from build123d import *

# Parameters (mm, degrees)
SKETCH1_R               = 6.35
BOSS_EXTRUDE1_DEPTH     = 25.4
SKETCH2_R               = 2.5
CUT_EXTRUDE1_DEPTH      = 12.7
SKETCH3_R               = 3.175
CUT_EXTRUDE2_DEPTH      = 12.7
CUT_EXTRUDE4_REACH      = 28.941
CUT_EXTRUDE4_END_RADIUS = 6.35
SKETCH4_R               = 1.3890625


with BuildPart() as part:
    # Sketch1 → Boss-Extrude1 (new body)
    with BuildSketch(Plane.XY):
        Circle(SKETCH1_R)
    extrude(amount=BOSS_EXTRUDE1_DEPTH)

    # Sketch2 → Cut-Extrude1 (cut)
    with BuildSketch(Plane.XY.offset(25.4)):
        Circle(SKETCH2_R)
    extrude(amount=-CUT_EXTRUDE1_DEPTH, mode=Mode.SUBTRACT)

    # Sketch3 → Cut-Extrude2 (cut)
    with BuildSketch(Plane(origin=(0, 0, 0), x_dir=(-1, 0, 0), z_dir=(0, 0, -1))):
        Circle(SKETCH3_R)
    extrude(amount=-CUT_EXTRUDE2_DEPTH, mode=Mode.SUBTRACT)

    # Cut-Extrude4: up to this cylinder (the profile starts inside it)
    cut_extrude4_end = Plane(origin=(0, 0, 12.7), z_dir=(0, 0, -1)) * Cylinder(CUT_EXTRUDE4_END_RADIUS, 90.632, mode=Mode.PRIVATE)
    # Sketch4 → Cut-Extrude4 (cut, up to the surface)
    with BuildSketch(Plane(origin=(0, 0, 0), x_dir=(1, 0, 0), z_dir=(0, 1, 0)), mode=Mode.PRIVATE) as cut_extrude4_sk1:
        with Locations(Location((0, -22.225, 0), (0, 0, 270))):
            Circle(SKETCH4_R)
    cut_extrude4_tool1 = extrude(cut_extrude4_sk1.sketch, amount=-CUT_EXTRUDE4_REACH, mode=Mode.PRIVATE) & cut_extrude4_end
    add(cut_extrude4_tool1.solids().sort_by_distance((0, 0, 22.225))[0], mode=Mode.SUBTRACT)
    # Sketch4 → Cut-Extrude4 (cut, up to the surface)
    with BuildSketch(Plane(origin=(0, 0, 0), x_dir=(1, 0, 0), z_dir=(0, 1, 0)), mode=Mode.PRIVATE) as cut_extrude4_sk2:
        with Locations(Location((0, -3.175, 0), (0, 0, 270))):
            Circle(SKETCH4_R)
    cut_extrude4_tool2 = extrude(cut_extrude4_sk2.sketch, amount=-CUT_EXTRUDE4_REACH, mode=Mode.PRIVATE) & cut_extrude4_end
    add(cut_extrude4_tool2.solids().sort_by_distance((0, 0, 3.175))[0], mode=Mode.SUBTRACT)


solid = part.part
Check sheet for the modelled part. Datum: model origin and axes. Units: mm. A direction names the side the tool comes from. Round coordinates to 2 decimals unless told otherwise and drop trailing zeros. Loops run counter-clockwise (first coordinate to the right, second up) from the corner with the lowest first, then second, coordinate; pieces in that order, holes last. Notation, with made-up numbers: M -25.5,70 L 3.5,70 A16 ccw 3.5,89 Z; hole C 59.5,-15.5 d10. An arc over 180 degrees is marked long. One line per question, with ' | ' between items. Start each with the question number.
Item 1: Section check C-C (z = 8.5). Record the boundary of the cut face in (x, y) (3 decimals).
Item 2: Section check A-A (y = 0). Record the boundary of the cut face in (x, z) (3 decimals).
Item 3: Gauge pin test, flat ends, axial feed: pin 1 Ø1.5 at (y, z) = (-4, 21.5) entering from -X; pin 2 Ø4 at (x, y) = (0, 0) entering from -Z; pin 3 Ø2 at (y, z) = (-3.5, 6) entering from -X. Record the tip position at first contact, or that the pin passes through.
Item 4: Section check B-B (x = 0). Record the boundary of the cut face in (y, z) (3 decimals), and give its area (3 significant figures).
Item 5: Set-up check for faces 1 (the face through (-2, 3, 0)), 2 (the face through (0.42, -4.19, 23.55)), 3 (the face through (0, -3, 12.7)): record each of +Z, -Z, +X, -X, +Y, -Y from which the full face is reachable in a straight line by a thin tool's end or side.
Item 6: Scan lines: probe 1 along Z at (x, y) = (0, -4); probe 2 along Y at (x, z) = (0, 18); probe 3 along Y at (x, z) = (0, 5.75) (3 decimals). Record each from-to range of solid material in increasing order.
Item 7: Release check for a two-part mould opening along Y. For faces 4 (the face through (-0.33, 2.48, 19.14)), 5 (the face through (-1.38, -6.2, 12.52)), 6 (the face through (0.41, 3.15, 6.26)), 7 (the face through (0.42, -4.58, 4.5)) record: released by +Y, released by -Y, zero draft, split by the parting line, or undercut.
Item 8: Section check D-D (x = -5.5). Record the boundary of the cut face in (y, z), and give its area (3 significant figures).
Worked out:
1) outline: C 0,0 d12.7; hole C 0,0 d6.35
2) outline: M -6.35,0 L -3.175,0 L -3.175,12.7 L -2.5,12.7 L -2.5,25.4 L -6.35,25.4 Z; M 2.5,12.7 L 3.175,12.7 L 3.175,0 L 6.35,0 L 6.35,25.4 L 2.5,25.4 Z
3) pin 1: x = -5.46 | pin 2: through | pin 3: x = -5.84
4) outline: M -6.35,0 L -3.175,0 L -3.175,1.786 L -6.35,1.786 Z; M -6.35,4.564 L -3.175,4.564 L -3.175,12.7 L -2.5,12.7 L -2.5,20.836 L -6.35,20.836 Z; M -6.35,23.614 L -2.5,23.614 L -2.5,25.4 L -6.35,25.4 Z; M 2.5,12.7 L 3.175,12.7 L 3.175,0 L 6.35,0 L 6.35,25.4 L 2.5,25.4 Z | area: 159 mm^2
5) face 1: -Z, +X, -X, +Y, -Y | face 2: -Y | face 3: -Z
6) probe 1: 0 to 1.79, 4.56 to 20.84, 23.61 to 25.4 | probe 2: -6.35 to -2.5, 2.5 to 6.35 | probe 3: -6.35 to -3.175, 3.175 to 6.35
7) face 4: undercut | face 5: split by the parting line | face 6: undercut | face 7: zero draft
8) outline: M -3.17,0 L 3.17,0 L 3.17,25.4 L -3.17,25.4 Z | area: 161 mm^2
